The model under review builds one solid part; all positions refer to its coordinate system, in mm. A direction names the side the tool comes from. Give positions to 0.01 mm unless a question says otherwise; leave off trailing zeros. Order: outer loops, then holes, each group sorted by start corner. A loop starts at its lowest first (then second) coordinate and runs counter-clockwise, first axis right, second up. Notation, with made-up numbers: (-20.75, 47) - (8.25, 47) arc R20 ccw to (8.25, 70) - close; hole circle Ø5 at (-18.75, 61.25). An arc over 180 degrees is marked (long way). Put each result on its own line as item: value.
```python
from build123d import *

# Parameters (mm, degrees)
SMUSSO1_SIZE = 1


with BuildPart() as part:
    # Schizzo1 → Rivoluzione1 (revolve)
    with BuildSketch(Plane.XY, mode=Mode.PRIVATE) as rivoluzione1_sk:
        Polygon((15.938425382, 0), (15.938425382, 2), (20.838425382, 2), (20.838425382, 7.5), (20.438425382, 7.5), (20.438425382, 9.47), (9.438425382, 9.47), (9.438425382, 7.5), (8.838425382, 7.5), (8.838425382, 4), (0.088425382, 4), (0.088425382, 3.68), (-1.161574618, 3.68), (-1.161574618, 4), (-11.161574618, 4), (-11.161574618, 0), align=None)
    revolve(rivoluzione1_sk.sketch.rotate(Axis((-12.465922444, 0, 0), (1, 0, 0)), 90), axis=Axis((-12.465922444, 0, 0), (1, 0, 0)))

    # Smusso1
    smusso1_edges = [part.edges().sort_by_distance(p)[0] for p in [
        (-11.161574618, 0, -4),
    ]]
    chamfer(smusso1_edges, length=SMUSSO1_SIZE)


solid = part.part
```
(1) Take a section at C-C, the plane x = -0.5. Write out the cut boundary in (y, z).
The answers:
outline: circle Ø7.36 at (0, 0)
(2) Take a section at B-B, the plane y = 5.5. Write out the cut boundary in (x, z).
The answers:
outline: (8.84, -5.1) - (9.44, -5.1) - (9.44, -7.71) - (20.44, -7.71) - (20.44, -5.1) - (20.84, -5.1) - (20.84, 5.1) - (20.44, 5.1) - (20.44, 7.71) - (9.44, 7.71) - (9.44, 5.1) - (8.84, 5.1) - close
(3) Clearance check with flat-ended pins moving along their axes: pin 1 Ø1.5 at (x, y) = (1.5, -1.5) entering from +Z; pin 2 Ø2 at (x, y) = (15, 2.5) entering from -Z; pin 3 Ø4 at (x, y) = (8.5, 5.5) entering from -Z. State where each tip first meets the part, or that it passes through.
The answers:
pin 1: z = 3.93
pin 2: z = -9.35
pin 3: z = -8.7
(4) For faces 1 (the cylindrical face through (9.134, -6.324, 4.032)), 2 (the cylindrical face through (-0.55, -3.65, -0.48)), 3 (the flat face through (-11.162, 0, 0)), 4 (the cylindrical face through (18, 2, 0)), list the 3-axis set-ups (+Z, -Z, +X, -X, +Y, -Y) from which the entire face can be reached by the end or side of a thin tool; tool diameter is ignored.
The answers:
face 1: -X
face 2: none
face 3: +Z, -Z, -X, +Y, -Y
face 4: +X
(5) Wall thickness on L1, parallel to Y at x = 19.3, z = 0; L2, parallel to X at y = 1.25, z = 6.5; L3, parallel to X at y = -8, z = -1.25: over which ranges is each line inside the solid? List them lowest first.
The answers:
L1: -9.47 to -2, 2 to 9.47
L2: 8.84 to 20.84
L3: 9.44 to 20.44
(6) The part is to be moulded in two halves that separate along Z. For faces 5 (the cylindrical face through (-5.725, 3.905, -0.867)), 6 (the flat face through (20.838, 2, -2)), 7 (the flat face through (15.938, 0, 0)), say which applies: pulls with the +Z half, pulls with the -Z half, needs draft (parallel to the pull), parting line crosses it, or undercut.
The answers:
face 5: parting line crosses it
face 6: needs draft
face 7: undercut
(7) Take a section at D-D, the plane z = -6.5. Write out the cut boundary in (x, y).
The answers:
outline: (8.84, -3.74) - (9.44, -3.74) - (9.44, -6.89) - (20.44, -6.89) - (20.44, -3.74) - (20.84, -3.74) - (20.84, 3.74) - (20.44, 3.74) - (20.44, 6.89) - (9.44, 6.89) - (9.44, 3.74) - (8.84, 3.74) - close
